```python
from build123d import *

# Parameters (mm, degrees)
SKETCH1_W           = 72
SKETCH1_H           = 35
SKETCH1_R           = 5.100000000000001
BOSS_EXTRUDE1_DEPTH = 10
FILLET1_R           = 12
SKETCH3_W           = 4.999999999999998
SKETCH3_H           = 4
CUT_EXTRUDE1_DEPTH  = 75.00000000000003
BOSS_EXTRUDE2_DEPTH = 6.5
BOSS_EXTRUDE3_DEPTH = 6.5
FILLET2_R           = 15
BOSS_EXTRUDE4_DEPTH = 5


with BuildPart() as part:
    # Sketch1 → Boss-Extrude1 (new body)
    with BuildSketch(Plane(origin=(0, 0, 0), x_dir=(1, 0, 0), z_dir=(0, 1, 0))):
        Rectangle(SKETCH1_W, SKETCH1_H)
        with Locations(Location((24, -5.500000000000002, 0), (0, 0, 270))):
            Circle(SKETCH1_R, mode=Mode.SUBTRACT)
        with Locations(Location((-24, -5.500000000000002, 0), (0, 0, 90))):
            Circle(SKETCH1_R, mode=Mode.SUBTRACT)
    extrude(amount=BOSS_EXTRUDE1_DEPTH)

    # Fillet1
    fillet1_edges = [part.edges().sort_by_distance(p)[0] for p in [
        (36.00000000000001, 5, 17.5),
        (-35.99999999999999, 5, 17.5),
    ]]
    fillet(fillet1_edges, radius=FILLET1_R)

    # Sketch3 → Cut-Extrude1 (cut)
    with BuildSketch(Plane.ZY.offset(35.99999999999999)):
        with Locations((-15, 8)):
            Rectangle(SKETCH3_W, SKETCH3_H)
    extrude(amount=-CUT_EXTRUDE1_DEPTH, mode=Mode.SUBTRACT)



with BuildPart() as body_2:
    # Sketch6 → Boss-Extrude2 (new, symmetric)
    with BuildSketch(Plane(origin=(0, 0, -12.5), x_dir=(-1, 0, 0), z_dir=(0, 0, -1))):
        with BuildLine():
            ThreePointArc((-15, 60), (-10.606601717798338, 49.393398282201915), (-3.4915e-13, 45))
            Line((0, 45), (0, 54))
            ThreePointArc((-1.4499e-13, 54), (-5.999999999999999, 60), (-1.4485e-13, 66))
            Line((0, 66), (0, 75))
            ThreePointArc((9.2e-16, 75), (-10.606601717798211, 70.60660171779821), (-15, 60))
        make_face()
        with BuildLine():
            Line((0, 54), (0, 45))
            ThreePointArc((-3.4915e-13, 45), (10.606601717798089, 49.39339828220166), (15, 59.99999999999999))
            ThreePointArc((15, 60), (10.606601717798213, 70.60660171779821), (4.25e-15, 75))
            Line((0, 75), (0, 66))
            ThreePointArc((-1.4485e-13, 66), (4.242640687119233, 64.24264068711933), (5.999999999999999, 60))
            ThreePointArc((5.999999999999999, 60), (4.242640687119235, 55.757359312880666), (-1.4499e-13, 54))
        make_face()
    extrude(amount=BOSS_EXTRUDE2_DEPTH, both=True)


with BuildPart() as part_1:
    add(part.part)

    add(body_2.part)  # Boss-Extrude3 merges body 2
    # Sketch6_3 → Boss-Extrude3 (add)
    with BuildSketch(Plane(origin=(0, 0, -12.5), x_dir=(-1, 0, 0), z_dir=(0, 0, -1))):
        with BuildLine():
            Line((-15, 10), (0, 10))
            Line((0, 10), (0, 45))
            ThreePointArc((-3.4915e-13, 45), (-10.606601717798338, 49.393398282201915), (-15, 60))
            Line((-15, 60), (-15, 10))
        make_face()
        with BuildLine():
            Line((0, 45), (0, 10))
            Line((0, 10), (15, 10))
            Line((15, 10), (15, 60))
            ThreePointArc((15, 59.99999999999999), (10.606601717798089, 49.39339828220166), (-3.4915e-13, 45))
        make_face()
    extrude(amount=-BOSS_EXTRUDE3_DEPTH)

    # Fillet2
    fillet2_edges = [part_1.edges().sort_by_distance(p)[0] for p in [
        (-15, 10, -9.25),
        (15, 10, -9.25),
    ]]
    fillet(fillet2_edges, radius=FILLET2_R)

    # Sketch7 → Boss-Extrude4 (add, symmetric)
    with BuildSketch(Plane(origin=(0, 0, 0), x_dir=(0, 0, -1), z_dir=(1, 0, 0))):
        Polygon((-17.5, 10), (6.000000000000002, 10), (6.000000000000001, 50), align=None)
    extrude(amount=BOSS_EXTRUDE4_DEPTH, both=True)


solid = part_1.part
```
Work out the finished part from the listing and answer in its coordinate system (mm). A direction names the side the tool comes from. Coordinates: 2 decimals unless noted, no trailing zeros. Write each loop counter-clockwise with the first axis right and the second up, starting at its lowest first coordinate (ties: lowest second). Pieces come first, ordered by that corner, then holes.
Q1. Determine the mould class of faces 5 (the face through (-1, 6, -15)), 6 (the face through (0, 54, -13)), 7 (the face through (15, 43, -9)), 8 (the face through (17, 10, 6)) for opening direction Y: released by +Y, released by -Y, zero draft, split by the parting line, or undercut.
Q2. A cutting plane is placed at D-D, the plane x = -12. Give the vertices of the cut face in (y, z), then the cut area to 4 significant figures.
Q3. Find the intervals of material crossed by line 1 (X direction, y = 3, z = 5); line 2 (Y direction, x = 28, z = -0.5); line 3 (Z direction, x = -27, y = 4.5), in increasing order.
Q4. A cutting plane is placed at C-C, the plane z = 8.5. Give the vertices of the cut face in (x, y), then the cut area to 3 significant figures.
Q5. A cutting plane is placed at B-B, the plane x = -28. Give the vertices of the cut face in (y, z), then the cut area to 3 significant figures.
Q6. Each of these flat-tipped pins is pushed along its axis until it touches: pin 1 Ø13.5 at (x, z) = (-24, 5.5) entering from -Y; pin 2 Ø7 at (y, z) = (39.5, -10) entering from +X; pin 3 Ø4 at (x, z) = (15, -15) entering from +Y; pin 4 Ø12 at (y, z) = (22, 3.5) entering from -X. Where does it stop, or does it pass through?
Q7. Which of the six approach directions +Z, -Z, +X, -X, +Y, -Y give full straight-line access (tool end or side, diameter ignored) to faces 1 (the face through (-0.66, 74.985, -14.035)), 2 (the face through (-1, 3, -17.5)), 3 (the face through (-17, 10, 6)), 4 (the face through (5, 21, 1))?
Q8. A cutting plane is placed at A-A, the plane z = -15. Give the vertices of the cut face in (x, y), then the cut area to 3 significant figures.
Findings below:
1. face 5: undercut
1. face 6: undercut
1. face 7: zero draft
1. face 8: released by +Y
2. outline: (0, -17.5) - (6, -17.5) - (6, -12.5) - (51, -12.5) - (51, -19) - (69, -19) - (69, -6) - (10, -6) - (10, 17.5) - (0, 17.5) - close
2. area: 830.5 mm2
3. line 1: x = -36 to -29.08, -18.92 to 18.92, 29.08 to 36
3. line 2: y = 0 to 10
3. line 3: z = -17.5 to 1.38, 9.62 to 17.12
4. outline: (-35.62, 0) - (-28.12, 0) - (-28.12, 10) - (-35.62, 10) - close; (-19.88, 0) - (19.88, 0) - (19.88, 10) - (5, 10) - (5, 25.32) - (-5, 25.32) - (-5, 10) - (-19.88, 10) - close; (28.12, 0) - (35.62, 0) - (35.62, 10) - (28.12, 10) - close
4. area: 701 mm2
5. outline: (0, -17.5) - (6, -17.5) - (6, -12.5) - (10.13, -12.5) - (10.13, -6) - (10, -6) - (10, 2.34) - (0, 2.34) - close; (0, 8.66) - (10, 8.66) - (10, 16.81) - (0, 16.81) - close
5. area: 261 mm2
6. pin 1: stops at y = 0
6. pin 2: stops at x = 15
6. pin 3: stops at y = 67.48
6. pin 4: stops at x = -5
7. face 1: -Z
7. face 2: -Z, +X, -X, -Y
7. face 3: +Z, -X, +Y
7. face 4: +Z, +X, +Y
8. outline: (-36, 0) - (36, 0) - (36, 6) - (-36, 6) - close; circle Ø30 at (0, 60); hole circle Ø12 at (0, 60)
8. area: 1,030 mm2
